Build history of the part. All positions in model axes, mm. A direction names the side the tool comes from. Give positions to 0.01 mm unless a question says otherwise; leave off trailing zeros. Order: outer loops, then holes, each group sorted by start corner. A loop starts at its lowest first (then second) coordinate and runs counter-clockwise, first axis right, second up. Notation, with made-up numbers: M -16,8.25 L -3,8.25 A20 cw -3,46.25 Z; hole C -10,-14 d2. An arc over 180 degrees is marked long. One line per item, written item: value. Start each with the question number.
from build123d import *

# Parameters (mm, degrees)
EXTRUDE_DEPTH                     = 40
EXTRUDE_ONTO_WIRE_PLACEMENT_ANGLE = -3e-06


with BuildPart() as part:
    # Wire as drawn → Extrude (new)
    with BuildSketch(Plane.XY):
        Polygon((0, 0), (16, 0), (16, 16), (14.5, 16), (14.5, 3), (11.5, 3), (11.5, 16), (10, 16), (10, 3), (6, 3), (6, 16), (4.5, 16), (4.5, 3), (1.5, 3), (1.5, 16), (0, 16), align=None)
    extrude(amount=EXTRUDE_DEPTH)


with BuildPart() as part_1:
    # Extrude onto Wire placement: moved
    add(part.part.moved(Location((3.622236, 2.417496, 0))).rotate(Axis((3.622236, 2.417496, 0), (0, 0, 1)), EXTRUDE_ONTO_WIRE_PLACEMENT_ANGLE))


solid = part_1.part
1) Slice it at C-C (x = 11.25). List the corners of the cut face in (y, z), plus the area to 3 significant figures.
2) Pull direction X, two halves, no side cores. Call faces 1 (the flat face through (7, 5.417, 20)), 2 (the flat face through (14, 18.417, 20)), 3 (the flat face through (19.622, 10, 20)): pulls with the +X half, pulls with the -X half, needs draft (parallel to the pull), parting line crosses it, or undercut.
3) Slice it at A-A (y = 11.5). List the corners of the cut face in (x, z), plus the area to 3 significant figures.
4) Drill centre lines: line 1 (X direction, y = 6, z = 20.5); line 2 (Y direction, x = 11.25, z = 32). Where is each one in solid material? Low to high.
5) Tool access for faces 4 (the flat face through (17, 5.417, 20)), 5 (the flat face through (9, 18.417, 20)): list every direction of +Z, -Z, +X, -X, +Y, -Y with a clear straight run to the whole face (end or side of a thin tool).
6) Slice it at B-B (z = 22.5). List the corners of the cut face in (x, y).
7) Drop a flat-ended pin along its axis: P1, Ø2, axis at x = 12, z = 10, coming from the +Y side. Give the stop position or say it passes through.
Results list:
1. outline: M 2.42,0 L 5.42,0 L 5.42,40 L 2.42,40 Z
1. area: 120 mm²
2. face 1: undercut
2. face 2: needs draft
2. face 3: pulls with the +X half
3. outline: M 3.62,0 L 5.12,0 L 5.12,40 L 3.62,40 Z; M 8.12,0 L 9.62,0 L 9.62,40 L 8.12,40 Z; M 13.62,0 L 15.12,0 L 15.12,40 L 13.62,40 Z; M 18.12,0 L 19.62,0 L 19.62,40 L 18.12,40 Z
3. area: 240 mm²
4. line 1: x = 3.62 to 5.12, 8.12 to 9.62, 13.62 to 15.12, 18.12 to 19.62
4. line 2: y = 2.42 to 5.42
5. face 4: +Z, -Z, +Y
5. face 5: +Z, -Z, +X, -X, +Y
6. outline: M 3.62,2.42 L 19.62,2.42 L 19.62,18.42 L 18.12,18.42 L 18.12,5.42 L 15.12,5.42 L 15.12,18.42 L 13.62,18.42 L 13.62,5.42 L 9.62,5.42 L 9.62,18.42 L 8.12,18.42 L 8.12,5.42 L 5.12,5.42 L 5.12,18.42 L 3.62,18.42 Z
7. P1: stops at y = 5.42
